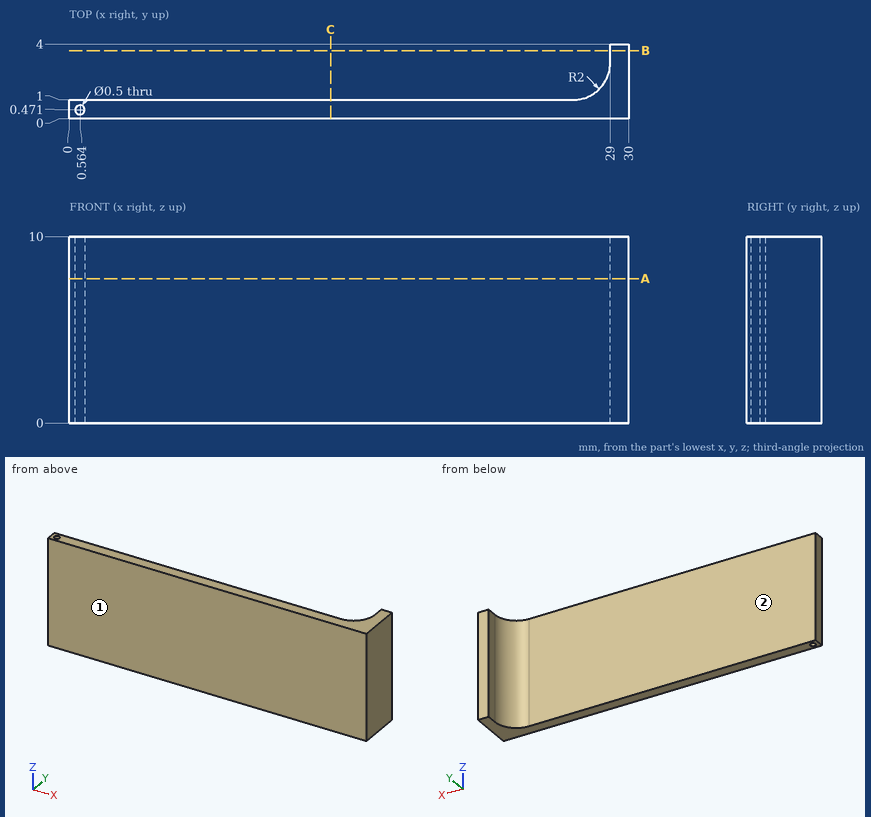
Geometry check sheet. Reference: drawing and pictorial views, mm from the part's lowest x, y, z. A direction names the side the tool comes from. Give positions to 0.01 mm unless a question says otherwise; leave off trailing zeros. Loops run counter-clockwise (first coordinate to the right, second up) from the corner with the lowest first, then second, coordinate; pieces in that order, holes last. Notation, with made-up numbers: (69.25, 67.5) -> (82.25, 67.5) arc R30 cw to (82.25, 89.5) -> close; hole circle Ø1 at (-33.75, -35). An arc over 180 degrees is marked (long way). Answer in a Markdown table with one row per item. Add a question column.
1) Cross-section at C-C on x = 14. Record the boundary of the cut face in (y, z).
2) Set-up check for the marked faces 1 and 2: record each of +Z, -Z, +X, -X, +Y, -Y from which the full face is reachable in a straight line by a thin tool's end or side.
3) Material ranges on probe 1 along Y at (x, z) = (23.75, 9.75); probe 2 along X at (y, z) = (3, 0.75); probe 3 along X at (y, z) = (2.15, 3.5), recorded low to high. Write a range as from..to.
4) Gauge pin test, flat ends, axial feed: P1, Ø3, axis at x = 13, z = 7.5, coming from the +Y side; P2, Ø1.1, axis at y = 3.5, z = 6, coming from the -X side. Record the tip position at first contact, or that the pin passes through.
5) Cross-section at A-A on z = 7.75. Record the boundary of the cut face in (x, y).
6) Cross-section at B-B on y = 3.65. Record the boundary of the cut face in (x, z), and give its area (3 significant figures).
Outcome:
| question | item | result |
|---|---|---|
| 1 | outline | (0, 0) -> (1, 0) -> (1, 10) -> (0, 10) -> close |
| 2 | face 1 | +Z, -Z, +X, -X, -Y |
| 2 | face 2 | +Z, -Z, -X, +Y |
| 3 | probe 1 | y = 0..1 |
| 3 | probe 2 | x = 29..30 |
| 3 | probe 3 | x = 28.81..30 |
| 4 | P1 | stops at y = 1 |
| 4 | P2 | stops at x = 29 |
| 5 | outline | (0, 0) -> (30, 0) -> (30, 4) -> (29, 4) -> (29, 3) arc R2 cw to (27, 1) -> (0, 1) -> close; hole circle Ø0.5 at (0.56, 0.47) |
| 6 | outline | (29, 0) -> (30, 0) -> (30, 10) -> (29, 10) -> close |
| 6 | area | 10.0 mm^2 |
